CAD build for the part. Positions are in the model's coordinates, mm. A direction names the side the tool comes from. Round coordinates to 2 decimals unless told otherwise and drop trailing zeros. Order: outer loops, then holes, each group sorted by start corner. A loop starts at its lowest first (then second) coordinate and runs counter-clockwise, first axis right, second up. Notation, with made-up numbers: (7, 56) - (32, 56) arc R34 cw to (32, 94) - close; hole circle Ø1 at (71.25, 67.25). An arc over 180 degrees is marked (long way). Write item = value, one per line.
from build123d import *

# Parameters (mm, degrees)
F1_DEPTH = 2


with BuildPart() as f1:
    # F0 (on Front) → F1 (new body)
    with BuildSketch(Plane.XZ):
        with BuildLine():
            Line((-124.6721289065, 66.9943112569), (-124.6721289065, -3.1820335149))
            add(Edge.make_bspline(
                [(-108.7886020541, -16.6170091142), (-115.0603290285, -12.3232285742), (-120.2999981868, -7.7183339998), (-124.6721289065, -3.1820335149)],
                knots=[0.4585261262, 0.4585261262, 0.4585261262, 0.4585261262, 0.6354781501, 0.6354781501, 0.6354781501, 0.6354781501], degree=3))
            Line((-108.7886020541, -16.6170091142), (-108.7886020541, 66.9943112569))
            Line((-108.7886020541, 66.9943112569), (-124.6721289065, 66.9943112569))
        make_face()
        with BuildLine():
            add(Edge.make_bspline(
                [(-142.2094079373, 80.4314068878), (-130.2931281445, 110.3476141939), (-98.2848527548, 116.0134827146), (-35.7470019427, 114.8680118272)],
                knots=[0, 0, 0, 0, 1, 1, 1, 1], degree=3))
            ThreePointArc((-142.2094079373, 80.4314068878), (-146.3504948166, 50.5368703201), (-142.0856537936, 20.6597377906))
            add(Edge.make_bspline(
                [(-124.6721289065, -3.1820335149), (-133.6787350082, 6.1627629347), (-139.0038412424, 15.2164724191), (-142.0856537936, 20.6597377906)],
                knots=[0.6354781501, 0.6354781501, 0.6354781501, 0.6354781501, 1, 1, 1, 1], degree=3))
            Line((-124.6721289065, -3.1820335149), (-124.6721289065, 66.9943112569))
            Line((-124.6721289065, 66.9943112569), (-108.7886020541, 66.9943112569))
            Line((-108.7886020541, 66.9943112569), (-108.7886020541, -16.6170091142))
            add(Edge.make_bspline(
                [(-36.381947872, -37.122189497), (-69.3556272485, -36.7804960017), (-92.5370180869, -27.743248389), (-108.7886020541, -16.6170091142)],
                knots=[0, 0, 0, 0, 0.4585261262, 0.4585261262, 0.4585261262, 0.4585261262], degree=3))
            add(Edge.make_bspline(
                [(-36.381947872, -37.122189497), (47.0810634374, -38.6126036396), (61.6125640752, -9.5495949141), (59.2237142208, 33.6754252563)],
                knots=[0, 0, 0, 0, 1, 1, 1, 1], degree=3))
            Line((59.2237142208, 33.6754252563), (59.2237142208, 42.0407210837))
            add(Edge.make_bspline(
                [(-35.7470019427, 114.8680118272), (4.2317536953, 114.8997140476), (50.434487808, 96.2695801058), (59.2237142208, 42.0407210837)],
                knots=[0, 0, 0, 0, 1, 1, 1, 1], degree=3))
        make_face()
        with BuildLine():
            Line((-65.2386816857, 47.185676674), (-50.5756217741, 84.2391779074))
            Line((-50.5756217741, 84.2391779074), (-21.8579741833, 84.2391779074))
            Line((-21.8579741833, 84.2391779074), (-7.197354984, 50.0167762288))
            Line((-7.197354984, 50.0167762288), (-7.197354984, 28.1597529901))
            ThreePointArc((-7.197354984, 28.1597529901), (-36.2556737781, 0.0750783929), (-65.2386816857, 28.237466271))
            Line((-65.2386816857, 28.237466271), (-65.2386816857, 47.185676674))
        make_face(mode=Mode.SUBTRACT)
    extrude(amount=F1_DEPTH)


solid = f1.part
(1) Probe line 1 along X through (y, z) = (-0.4, 23); line 2 along Z through (x, y) = (-33, -0.6); line 3 along X through (y, z) = (-0.05, 53). List the from-to ranges inside material, lowest first.
Solved:
line_1 = -142.73 to -64.6, -7.83 to 59.43
line_2 = -37.17 to 0.25, 84.24 to 114.84
line_3 = -146.33 to -62.94, -8.48 to 56.82
(2) Drop flat-ended pins along their axis: pin 1 (0.6 mm diameter, centred on y = -0.5, z = 36, fed in from +X); pin 2 (1 mm diameter, centred on y = -1, z = -15.5, fed in from -X). Give the stop position or say it passes through.
Solved:
pin_1 = 59.22
pin_2 = -111.08
(3) Pull direction Z, two halves, no side cores. Call faces 1 (the flat face through (-14.63, -0.99, 67.37)), 2 (the cylindrical face through (-146.35, -0.99, 50.96)), 3 (the flat face through (-67, 0, 40)), 4 (the cylindrical face through (-35.63, -0.99, 0.08)): released by +Z, released by -Z, zero draft, split by the parting line, or undercut.
Solved:
face_1 = undercut
face_2 = split by the parting line
face_3 = zero draft
face_4 = undercut
(4) Band-saw the part on A-A on z = 39. List the corners of the cut face in (x, y).
Solved:
outline = (-145.71, -2) - (-65.24, -2) - (-65.24, 0) - (-145.71, 0) - close; (-7.2, -2) - (59.22, -2) - (59.22, 0) - (-7.2, 0) - close
(5) Tool access for faces 5 (the flat face through (-58.01, -0.99, 65.45)), 6 (the flat face through (-67, -2, 40)): list every direction of +Z, -Z, +X, -X, +Y, -Y with a clear straight run to the whole face (end or side of a thin tool).
Solved:
face_5 = +Y, -Y
face_6 = +Z, -Z, +X, -X, -Y
